from build123d import *

# Parameters (mm, degrees)
SKETCH1_R           = 3.556
BOSS_EXTRUDE1_DEPTH = 76.2
SKETCH2_R           = 1.905
CUT_EXTRUDE1_DEPTH  = 6.604
SKETCH3_W           = 58.057716114
SKETCH3_H           = 2.54
SKETCH3_W_2         = 2.54
SKETCH3_H_2         = 26.67
SKETCH3_W_3         = 58.42
SKETCH3_H_3         = 15.24
BOSS_EXTRUDE2_DEPTH = 17.78
SKETCH4_W           = 6.858
SKETCH4_H           = 2.54
SKETCH4_W_2         = 2.54
SKETCH4_H_2         = 10.16
SKETCH4_H_3         = 18.288
BOSS_EXTRUDE3_DEPTH = 7.112
SKETCH5_R           = 1.905
CUT_EXTRUDE2_DEPTH  = 7.112


with BuildPart() as part:
    # Sketch1 → Boss-Extrude1 (new body)
    with BuildSketch(Plane.XY):
        with BuildLine():
            Line((-44.45, 6.096), (44.45, 6.096))
            ThreePointArc((44.45, 6.096), (50.546, 0), (44.45, -6.096))
            Line((44.45, -6.096), (-44.45, -6.096))
            ThreePointArc((-44.45, -6.096), (-50.546, 0), (-44.45, 6.096))
        make_face()
        with Locations((-44.45, 0)):
            Circle(SKETCH1_R, mode=Mode.SUBTRACT)
        with Locations((44.45, 0)):
            Circle(SKETCH1_R, mode=Mode.SUBTRACT)
    extrude(amount=BOSS_EXTRUDE1_DEPTH)

    # Sketch2 → Cut-Extrude1 (cut)
    with BuildSketch(Plane.XZ.offset(6.096)):
        with Locations((-9.144, 69.215)):
            Circle(SKETCH2_R)
        with Locations((27.051, 60.833)):
            Circle(SKETCH2_R)
        with Locations((-28.956, 69.215)):
            Circle(SKETCH2_R)
        with Locations((-28.956, 6.985)):
            Circle(SKETCH2_R)
        with Locations((-9.144, 6.985)):
            Circle(SKETCH2_R)
        with Locations((11.049, 60.833)):
            Circle(SKETCH2_R)
        with Locations((11.049, 15.367)):
            Circle(SKETCH2_R)
        with Locations((27.051, 15.367)):
            Circle(SKETCH2_R)
    extrude(amount=-CUT_EXTRUDE1_DEPTH, mode=Mode.SUBTRACT)

    # Sketch3 → Boss-Extrude2 (add)
    with BuildSketch(Plane(origin=(0, 6.096, 0), x_dir=(1, 0, 0), z_dir=(0, 1, 0))):
        with Locations((-0.181141943, -13.97)):
            Rectangle(SKETCH3_W, SKETCH3_H)
        with Locations((-27.94, -28.575)):
            Rectangle(SKETCH3_W_2, SKETCH3_H_2)
        with Locations((0, -43.18)):
            Rectangle(SKETCH3_W_3, SKETCH3_H)
        with Locations((27.577716114, -22.86)):
            Rectangle(SKETCH3_W_2, SKETCH3_H_3)
    extrude(amount=BOSS_EXTRUDE2_DEPTH)

    # Sketch4 → Boss-Extrude3 (add)
    with BuildSketch(Plane(origin=(0, 6.096, 0), x_dir=(1, 0, 0), z_dir=(0, 1, 0))):
        with Locations((-32.639, -43.18)):
            Rectangle(SKETCH4_W, SKETCH4_H)
        with Locations((-34.798, -57.658)):
            Rectangle(SKETCH4_W_2, SKETCH4_H_2)
        Polygon((36.068, -62.738), (33.528, -62.738), (-33.528, -62.738), (-36.068, -62.738), (-36.068, -65.278), (36.068, -65.278), align=None)
        with Locations((34.798, -53.594)):
            Rectangle(SKETCH4_W_2, SKETCH4_H_3)
        with Locations((32.639, -43.18)):
            Rectangle(SKETCH4_W, SKETCH4_H)
    extrude(amount=BOSS_EXTRUDE3_DEPTH)

    # Sketch5 → Cut-Extrude2 (cut)
    with BuildSketch(Plane(origin=(0, 6.096, 0), x_dir=(1, 0, 0), z_dir=(0, 1, 0))):
        with Locations((38.608, -60.96)):
            Circle(SKETCH5_R)
        with Locations((-38.608, -60.96)):
            Circle(SKETCH5_R)
        with Locations((-38.608, -15.24)):
            Circle(SKETCH5_R)
        with Locations((38.608, -15.24)):
            Circle(SKETCH5_R)
    extrude(amount=-CUT_EXTRUDE2_DEPTH, mode=Mode.SUBTRACT)


solid = part.part
Part model, mm, in its own coordinate system. A direction names the side the tool comes from. Give positions to 0.01 mm unless a question says otherwise; leave off trailing zeros. Order: outer loops, then holes, each group sorted by start corner. A loop starts at its lowest first (then second) coordinate and runs counter-clockwise, first axis right, second up. Notation, with made-up numbers: (-33, -18) - (-7, -18) arc R27 cw to (-7, 3) - close; hole circle Ø7 at (78.5, -26). An arc over 180 degrees is marked (long way). Use a Markdown table: item, result.
1) Flat gauge pins, fed straight in: P1, Ø0.8, axis at x = -35, y = 10, coming from the -Z side; P2, Ø1.9, axis at x = 38, z = 61, coming from the +Y side; P3, Ø6, axis at x = -38.608, z = 60.96, coming from the +Y side; P4, Ø6, axis at x = -7.5, y = 8.5, coming from the -Z side. Where does each tip first touch, or does it go through?
Checked values:
| item | result |
|---|---|
| P1 | z = 41.91 |
| P2 | y = -1.02 |
| P3 | y = 13.21 |
| P4 | z = 0 |
2) Saw through at A-A on z = 46.5. List the corners of the cut face in (x, y), plus the area to 3 significant figures.
Checked values:
| item | result |
|---|---|
| outline | (-44.45, -6.1) - (44.45, -6.1) arc R6.1 ccw to (44.45, 6.1) - (36.07, 6.1) - (36.07, 13.21) - (33.53, 13.21) - (33.53, 6.1) - (-44.45, 6.1) arc R6.1 ccw to start; hole circle Ø7.11 at (-44.45, 0); hole circle Ø7.11 at (44.45, 0) |
| area | 1,140 mm² |
3) Saw through at D-D on y = 16. List the corners of the cut face in (x, z).
Checked values:
| item | result |
|---|---|
| outline | (-29.21, 12.7) - (28.85, 12.7) - (28.85, 30.48) - (26.31, 30.48) - (26.31, 15.24) - (-26.67, 15.24) - (-26.67, 41.91) - (29.21, 41.91) - (29.21, 44.45) - (-29.21, 44.45) - close |
4) 3-axis set-ups, long thin cutter, end or side, ignore diameter. For faces 5 (the cylindrical face through (-40.51, 2.59, 15.16)), 6 (the flat face through (11, 0.508, 61)): which of +Z, -Z, +X, -X, +Y, -Y reach the whole face in a straight line?
Checked values:
| item | result |
|---|---|
| face 5 | +Y |
| face 6 | -Y |
5) Probe L1, parallel to Z at x = -12.5, y = 8; L2, parallel to X at y = -1.5, z = 51; L3, parallel to X at y = 10.5, z = 55. List the from-to ranges inside material, lowest first. Write a range as from..to.
Checked values:
| item | result |
|---|---|
| L1 | 12.7..15.24, 41.91..44.45, 62.74..65.28 |
| L2 | -50.36..-47.67, -41.23..41.23, 47.67..50.36 |
| L3 | -36.07..-33.53, 33.53..36.07 |
6) Two-plate mould, pull along Z, no slides. Class faces 1 (the flat face through (-36.068, 10, 59)), 2 (the cylindrical face through (12.866, -2.84, 15.939)), 3 (the flat face through (-1, 15, 12.7)), 4 (the flat face through (4, 15, 41.91)): +Z half, -Z half, draft (parallel to the pull), parting line (faces both ways), or undercut.
Checked values:
| item | result |
|---|---|
| face 1 | draft |
| face 2 | undercut |
| face 3 | -Z half |
| face 4 | undercut |
7) Saw through at C-C on x = -17. List the corners of the cut face in (y, z), plus the area to 3 significant figures.
Checked values:
| item | result |
|---|---|
| outline | (-6.1, 0) - (6.1, 0) - (6.1, 12.7) - (23.88, 12.7) - (23.88, 15.24) - (6.1, 15.24) - (6.1, 41.91) - (23.88, 41.91) - (23.88, 44.45) - (6.1, 44.45) - (6.1, 62.74) - (13.21, 62.74) - (13.21, 65.28) - (6.1, 65.28) - (6.1, 76.2) - (-6.1, 76.2) - close |
| area | 1,040 mm² |
8) Saw through at B-B on y = 7.5. List the corners of the cut face in (x, z).
Checked values:
| item | result |
|---|---|
| outline | (-36.07, 41.91) - (-29.21, 41.91) - (-29.21, 12.7) - (28.85, 12.7) - (28.85, 30.48) - (26.31, 30.48) - (26.31, 15.24) - (-26.67, 15.24) - (-26.67, 41.91) - (36.07, 41.91) - (36.07, 65.28) - (-36.07, 65.28) - (-36.07, 52.58) - (-33.53, 52.58) - (-33.53, 62.74) - (33.53, 62.74) - (33.53, 44.45) - (-36.07, 44.45) - close |
